```python
from build123d import *

# Parameters (mm, degrees)
BOSS_EXTRUDE1_DEPTH                           = 5
CBORE_FOR_M6_PAN_HEAD_MACHINE_SCREW1_AT_COUNT = 2
CBORE_FOR_M6_PAN_HEAD_MACHINE_SCREW1_AT_PITCH = 90
CBORE_FOR_M6_PAN_HEAD_MACHINE_SCREW1_2_COUNT  = 2
CBORE_FOR_M6_PAN_HEAD_MACHINE_SCREW1_2_PITCH  = 90
LPATTERN1_COUNT                               = 2
LPATTERN1_PITCH                               = 560
M5_CLEARANCE_HOLE1_AT_2_COUNT                 = 2
M5_CLEARANCE_HOLE1_AT_2_PITCH                 = 38.907056767
M5_CLEARANCE_HOLE1_AT_3_COUNT                 = 2
M5_CLEARANCE_HOLE1_AT_3_PITCH                 = 118.743434782
LPATTERN2_COUNT                               = 2
LPATTERN2_PITCH                               = 93


with BuildPart() as part:
    # Sketch1 → Boss-Extrude1 (new body)
    with BuildSketch(Plane.XY):
        with BuildLine():
            Line((-296.5, -120), (296.5, -120))
            ThreePointArc((296.5, -120), (299.328427125, -118.828427125), (300.5, -116))
            Line((300.5, -116), (300.5, 116))
            ThreePointArc((300.5, 116), (299.328427125, 118.828427125), (296.5, 120))
            Line((296.5, 120), (-296.5, 120))
            ThreePointArc((-296.5, 120), (-299.328427125, 118.828427125), (-300.5, 116))
            Line((-300.5, 116), (-300.5, -116))
            ThreePointArc((-300.5, -116), (-299.328427125, -118.828427125), (-296.5, -120))
        make_face()
    extrude(amount=BOSS_EXTRUDE1_DEPTH)

    # Sketch2 → CBORE for M6 Pan Head Machine Screw1 (revolve, cut)
    with BuildSketch(Plane(origin=(280.273194374, 0, 5), x_dir=(0, -1, 0), z_dir=(1, 0, 0))):
        Polygon((0, 0), (0, 6.982840043), (3.3, 5), (3.3, 4.625), (3.325, 4.6), (6.5, 4.6), (6.5, 0), align=None)
    cbore_for_m6_pan_head_machine_screw1 = revolve(axis=Axis((280.273194374, 0, 11.35), (0, 0, -1)), mode=Mode.SUBTRACT)

    # CBORE for M6 Pan Head Machine Screw1 at: CBORE for M6 Pan Head Machine Screw1 ×2
    with Locations(*[(0, i * CBORE_FOR_M6_PAN_HEAD_MACHINE_SCREW1_AT_PITCH, 0) for i in range(1, CBORE_FOR_M6_PAN_HEAD_MACHINE_SCREW1_AT_COUNT)]):
        add(cbore_for_m6_pan_head_machine_screw1, mode=Mode.SUBTRACT)

    # CBORE for M6 Pan Head Machine Screw1 2: CBORE for M6 Pan Head Machine Screw1 ×2
    with Locations(*[(0, -i * CBORE_FOR_M6_PAN_HEAD_MACHINE_SCREW1_2_PITCH, 0) for i in range(1, CBORE_FOR_M6_PAN_HEAD_MACHINE_SCREW1_2_COUNT)]):
        add(cbore_for_m6_pan_head_machine_screw1, mode=Mode.SUBTRACT)

    # LPattern1: CBORE for M6 Pan Head Machine Screw1 ×2
    with Locations(*[(-i * LPATTERN1_PITCH, 0, 0) for i in range(1, LPATTERN1_COUNT)]):
        add(cbore_for_m6_pan_head_machine_screw1, mode=Mode.SUBTRACT)

    # LPattern1 copy 1 sketch → LPattern1 copy 1 (revolve, cut)
    with BuildSketch(Plane(origin=(-279.726805626, 90, 5), x_dir=(0, -1, 0), z_dir=(1, 0, 0))):
        Polygon((0, 0), (0, 6.982840043), (3.3, 5), (3.3, 4.625), (3.325, 4.6), (6.5, 4.6), (6.5, 0), align=None)
    revolve(axis=Axis((-279.726805626, 90, 11.35), (0, 0, -1)), mode=Mode.SUBTRACT)

    # LPattern1 copy 2 sketch → LPattern1 copy 2 (revolve, cut)
    with BuildSketch(Plane(origin=(-279.726805626, -90, 5), x_dir=(0, -1, 0), z_dir=(1, 0, 0))):
        Polygon((0, 0), (0, 6.982840043), (3.3, 5), (3.3, 4.625), (3.325, 4.6), (6.5, 4.6), (6.5, 0), align=None)
    revolve(axis=Axis((-279.726805626, -90, 11.35), (0, 0, -1)), mode=Mode.SUBTRACT)

    # Sketch4 → M5 Clearance Hole1 (revolve, cut)
    with BuildSketch(Plane(origin=(-60.375010772, -63.419690337, 5), x_dir=(0, -1, 0), z_dir=(1, 0, 0))):
        Polygon((0, 0), (0, 6.652366702), (2.75, 5), (2.75, 0), align=None)
    m5_clearance_hole1 = revolve(axis=Axis((-60.375010772, -63.419690337, 11.35), (0, 0, -1)), mode=Mode.SUBTRACT)

    # M5 Clearance Hole1 at 2: M5 Clearance Hole1 ×2
    with Locations(*[(i * M5_CLEARANCE_HOLE1_AT_2_PITCH, 0, 0) for i in range(1, M5_CLEARANCE_HOLE1_AT_2_COUNT)]):
        add(m5_clearance_hole1, mode=Mode.SUBTRACT)

    # M5 Clearance Hole1 at 3: M5 Clearance Hole1 ×2
    with Locations(*[Vector(0.9999978769286347, 0.002060615981510638, 0) * (i * M5_CLEARANCE_HOLE1_AT_3_PITCH) for i in range(1, M5_CLEARANCE_HOLE1_AT_3_COUNT)]):
        add(m5_clearance_hole1, mode=Mode.SUBTRACT)

    # LPattern2: M5 Clearance Hole1 ×2
    with Locations(*[(0, i * LPATTERN2_PITCH, 0) for i in range(1, LPATTERN2_COUNT)]):
        add(m5_clearance_hole1, mode=Mode.SUBTRACT)

    # LPattern2 copy 1 sketch → LPattern2 copy 1 (revolve, cut)
    with BuildSketch(Plane(origin=(-21.467954006, 29.580309663, 5), x_dir=(0, -1, 0), z_dir=(1, 0, 0))):
        Polygon((0, 0), (0, 6.652366702), (2.75, 5), (2.75, 0), align=None)
    revolve(axis=Axis((-21.467954006, 29.580309663, 11.35), (0, 0, -1)), mode=Mode.SUBTRACT)

    # LPattern2 copy 2 sketch → LPattern2 copy 2 (revolve, cut)
    with BuildSketch(Plane(origin=(58.368171909, 29.824994283, 5), x_dir=(0, -1, 0), z_dir=(1, 0, 0))):
        Polygon((0, 0), (0, 6.652366702), (2.75, 5), (2.75, 0), align=None)
    revolve(axis=Axis((58.368171909, 29.824994283, 11.35), (0, 0, -1)), mode=Mode.SUBTRACT)


solid = part.part
```
Geometry check sheet. Reference: the model listing, model coordinates, mm. A direction names the side the tool comes from. Give positions to 0.01 mm unless a question says otherwise; leave off trailing zeros. Answer in a Markdown table with one row per item. Add a question column.
Q1. Mould release check, pull along X, two halves, no side actions. Record for faces 1 (the flat face through (-283, -92, 0.4)), 2 (the flat face through (-4, 2, 5)): pulls with the +X half, pulls with the -X half, needs draft (parallel to the pull), parting line crosses it, or undercut.
Q2. Material ranges on probe 1 along X at (y, z) = (-90, 0.2); probe 2 along Y at (x, z) = (-61, 0.65); probe 3 along X at (y, z) = (-90, 3.65), recorded low to high. Write a range as from..to.
Q3. Gauge pin test, flat ends, axial feed: pin 1 (10.5 mm diameter, centred on x = 277, y = 2, fed in from +Z); pin 2 (4 mm diameter, centred on x = -278, y = -87.5, fed in from +Z). Record the tip position at first contact, or that the pin passes through.
Q4. Tool access check on faces 3 (the flat face through (-4, 2, 0)), 4 (the flat face through (277, 88, 0.4)). Record the directions out of +Z, -Z, +X, -X, +Y, -Y that give a thin tool (end or side, any length) a straight path to the whole face; none if there is none.
Check values:
| question | item | result |
|---|---|---|
| 1 | face 1 | undercut |
| 1 | face 2 | needs draft |
| 2 | probe 1 | x = -300.5..-283.03, -276.43..276.97, 283.57..300.5 |
| 2 | probe 2 | y = -120..-66.1, -60.74..26.9, 32.26..120 |
| 2 | probe 3 | x = -300.5..-286.23, -273.23..273.77, 286.77..300.5 |
| 3 | pin 1 | stops at z = 5 |
| 3 | pin 2 | stops at z = 0.4 |
| 4 | face 3 | -Z, +X, -X, +Y, -Y |
| 4 | face 4 | +Z |
